Verification items for the finished model (mm, model axes). A direction names the side the tool comes from. Give positions to 0.01 mm unless a question says otherwise; leave off trailing zeros. Loops run counter-clockwise (first coordinate to the right, second up) from the corner with the lowest first, then second, coordinate; pieces in that order, holes last. Notation, with made-up numbers: (9, -33) - (34, -33) arc R13 ccw to (34, -10) - close; hole circle Ø6 at (-23.5, 43.5). An arc over 180 degrees is marked (long way). Put each result on its own line as item: value. Start each with the question number.
```python
from build123d import *

# Parameters (mm, degrees)
SKETCH_W        = 25
SKETCH_H        = 14
PAD_DEPTH       = 6
SKETCH001_R     = 3
POCKET_DEPTH    = 6
SKETCH002_R     = 1.55
POCKET001_DEPTH = 15
POCKET002_DEPTH = 5
FILLET_R        = 1


with BuildPart() as part:
    # Sketch → Pad (new body, symmetric)
    with BuildSketch(Plane.XY):
        Rectangle(SKETCH_W, SKETCH_H)
    extrude(amount=PAD_DEPTH, both=True)

    # Sketch001 → Pocket (cut)
    with BuildSketch(Plane.XY.offset(6)):
        with BuildLine():
            ThreePointArc((-2.2, -3.925557), (3.882654, 2.274863), (-4.5, 0))
            Line((-4.5, 0), (-4.5, -7))
            Line((-4.5, -7), (-2.2, -7))
            Line((-2.2, -7), (-2.2, -3.925557))
        make_face()
        Circle(SKETCH001_R, mode=Mode.SUBTRACT)
    extrude(amount=-POCKET_DEPTH, mode=Mode.SUBTRACT)

    # Sketch002 → Pocket001 (cut)
    with BuildSketch(Plane(origin=(0, 7, 0), x_dir=(-1, 0, 0), z_dir=(0, 1, 0))):
        with Locations((-8.5, 0)):
            Circle(SKETCH002_R)
        with Locations((8.5, 0)):
            Circle(SKETCH002_R)
    extrude(amount=-POCKET001_DEPTH, mode=Mode.SUBTRACT)

    # Sketch003 → Pocket002 (cut)
    with BuildSketch(Plane.XZ.offset(7)):
        Polygon((-5.75, -1.587713), (-5.75, 1.587713), (-8.5, 3.175426), (-11.25, 1.587713), (-11.25, -1.587713), (-8.5, -3.175426), align=None)
        Polygon((5.75, -1.587713), (8.5, -3.175426), (11.25, -1.587713), (11.25, 1.587713), (8.5, 3.175426), (5.75, 1.587713), align=None)
    extrude(amount=-POCKET002_DEPTH, mode=Mode.SUBTRACT)

    # Fillet
    fillet_edges = [part.edges().sort_by_distance(p)[0] for p in [
        (-2.2, -3.925557, 3),
    ]]
    fillet(fillet_edges, radius=FILLET_R)


solid = part.part
```
1) Section check C-C, the plane y = 5. Enter the section's corners in (x, z).
2) Scan lines: line 1 along Y through (x, z) = (0, 3.45); line 2 along X through (y, z) = (2.25, 4.75); line 3 along Y through (x, z) = (2.75, 2). Record each from-to range of solid material in increasing order. Write a range as from..to.
3) Section check D-D, the plane x = 0. Enter the section's corners in (y, z).
4) Draft check along Z on faces 1 (the face through (-4.5, -3, 3)), 2 (the face through (-11.25, -5, 0)), 3 (the face through (0, 5, 6)). Enter one of: pulls with the +Z half, pulls with the -Z half, needs draft (parallel to the pull), parting line crosses it, or undercut.
5) Set-up check for faces 4 (the face through (-2.2, -6, 3)), 5 (the face through (0, 0, -6)), 6 (the face through (9.86, -4.54, -2.39)), 7 (the face through (3.6, 2.7, 3)), 8 (the face through (0, -7, 0)): record each of +Z, -Z, +X, -X, +Y, -Y from which the full face is reachable in a straight line by a thin tool's end or side.
6) Section check A-A, the plane x = -8.75. Enter the section's corners in (y, z).
7) Section check B-B, the plane z = 4.75. Enter the section's corners in (x, y), plus the area to 3 significant figures.
8) Depth check by flat-ended pin: P1, Ø3, axis at x = 8.5, z = -1, coming from the -Y side. Enter the tip coordinate at first touch or a pass-through.
Results are:
1. outline: (-12.5, -6) - (12.5, -6) - (12.5, 6) - (-12.5, 6) - close; hole circle Ø3.1 at (-8.5, 0); hole circle Ø3.1 at (8.5, 0)
2. line 1: y = -7..-4.5, -3..3, 4.5..7
2. line 2: x = -12.5..-3.9, -1.98..1.98, 3.9..12.5
2. line 3: y = -7..-3.56, -1.2..1.2, 3.56..7
3. outline: (-7, -6) - (7, -6) - (7, 6) - (4.5, 6) - (4.5, 0) - (3, 0) - (3, 6) - (-3, 6) - (-3, 0) - (-4.5, 0) - (-4.5, 6) - (-7, 6) - close
4. face 1: needs draft
4. face 2: undercut
4. face 3: pulls with the +Z half
5. face 4: +Z, -Y
5. face 5: -Z, +X, -X, +Y, -Y
5. face 6: -Y
5. face 7: +Z
5. face 8: +Z, -Z, +X, -X, -Y
6. outline: (-7, -6) - (7, -6) - (7, -1.53) - (-2, -1.53) - (-2, -3.03) - (-7, -3.03) - close; (-7, 3.03) - (-2, 3.03) - (-2, 1.53) - (7, 1.53) - (7, 6) - (-7, 6) - close
7. outline: (-12.5, -7) - (-4.5, -7) - (-4.5, 0) arc R4.5 cw (long way) to (-0.98, -4.39) arc R1 ccw to (-2.2, -5.37) - (-2.2, -7) - (12.5, -7) - (12.5, 7) - (-12.5, 7) - close; circle Ø6 at (0, 0)
7. area: 305 mm2
8. P1: stops at y = -2
